```python
from build123d import *

# Parameters (mm, degrees)
F0_W      = 67.6028169692
F0_H      = 53.0741475523
F1_DEPTH  = 37.4
F2_R      = 11.3511276649
F2_R_2    = 7.9567380282
F3_DEPTH  = 6.7
F4_R      = 4.4090907082
F4_R_2    = 5.1686616875
F5_DEPTH  = 3.4
F7_DEPTH  = 2.1
F8_W      = 34.6914194524
F8_H      = 6.529385224
F9_DEPTH  = 4.6
F10_W     = 88.7872502208
F10_H     = 44.3032570183
F11_DEPTH = 87.7
F12_W     = 22.9829689488
F12_H     = 93.6014018953
F13_DEPTH = 18.4
F14_W     = 23.3173291199
F14_H     = 77.2590063095
F14_H_2   = 16.0102971315
F15_DEPTH = 18.6
F16_W     = 27.0305555314
F16_H     = 14.4476275891
F16_W_2   = 26.7750890926
F16_H_2   = 15.4520794749
F17_DEPTH = 103
F18_W     = 27.0305555314
F18_H     = 29.6849496663
F18_W_2   = 28.8268793374
F19_DEPTH = 10
F20_R     = 5


with BuildPart() as f1:
    # F0 (on Front) → F1 (new body)
    with BuildSketch(Plane.XZ):
        with Locations((1.2461747974, -5.0753373653)):
            Rectangle(F0_W, F0_H)
    extrude(amount=F1_DEPTH)

    # F2 (on face) → F3 (join)
    with BuildSketch(Plane.XZ.offset(37.4)):
        with Locations((-14.182465151, 1.8661138602)):
            Circle(F2_R)
        with Locations((17.3548590392, 0)):
            Circle(F2_R_2)
    extrude(amount=F3_DEPTH)

    # F4 (on face) → F5 (cut)
    with BuildSketch(Plane.XZ.offset(44.1)):
        with Locations((-14.182465151, 1.8661138602)):
            Circle(F4_R)
        with Locations((17.1402301639, 0)):
            Circle(F4_R_2)
    extrude(amount=-F5_DEPTH, mode=Mode.SUBTRACT)

    # F6 (on face) → F7 (cut)
    with BuildSketch(Plane.XZ.offset(37.4)):
        with BuildLine():
            add(Edge.make_bspline(
                [(-21.2736967951, -12.5029627234), (-17.6056978222, -10.7879533319), (1.7937398343, -27.2198277591), (39.0741519283, -6.345360962), (7.1844121531, -32.2427894232), (-23.5988764514, -26.0051011351), (-23.4195291506, -13.5062679776), (-21.2736967951, -12.5029627234)],
                knots=[0, 0, 0, 0, 0.217341047, 0.4323199028, 0.6402459683, 0.8728523496, 1, 1, 1, 1], degree=3))
        make_face()
    extrude(amount=-F7_DEPTH, mode=Mode.SUBTRACT)

    # F8 (on face) → F9 (join)
    with BuildSketch(Plane(origin=(0, 0, -31.6124111414), x_dir=(1, 0, 0), z_dir=(0, 0, -1))):
        with Locations((2.0386911929, 19.4482291117)):
            Rectangle(F8_W, F8_H)
    extrude(amount=F9_DEPTH)

    # F10 (on face) → F11 (join)
    with BuildSketch(Plane(origin=(0, 0, -36.2124111414), x_dir=(1, 0, 0), z_dir=(0, 0, -1))):
        with Locations((0.4012212157, 17.9098602384)):
            Rectangle(F10_W, F10_H)
    extrude(amount=F11_DEPTH)

    # F12 (on face) → F13 (join)
    with BuildSketch(Plane.YZ.offset(44.7948463261)):
        with Locations((-18.3663782664, -93.6325211078)):
            Rectangle(F12_W, F12_H)
    extrude(amount=F13_DEPTH)

    # F14 (on face) → F15 (join)
    with BuildSketch(Plane(origin=(-43.9924038947, 0, 0), x_dir=(0, -1, 0), z_dir=(-1, 0, 0))):
        with Locations((18.3590447996, -85.2829079866)):
            Rectangle(F14_W, F14_H)
        with Locations((18.3590447996, -131.9175597072)):
            Rectangle(F14_W, F14_H_2)
    extrude(amount=F15_DEPTH)

    # F16 (on face) → F17 (join)
    with BuildSketch(Plane(origin=(0, 0, -123.9124111414), x_dir=(1, 0, 0), z_dir=(0, 0, -1))):
        with Locations((-13.5152777657, 15.4278827831)):
            Rectangle(F16_W, F16_H)
        with Locations((22.6432844065, 15.930108726)):
            Rectangle(F16_W_2, F16_H_2)
    extrude(amount=F17_DEPTH)

    # F18 (on face) → F19 (join)
    with BuildSketch(Plane(origin=(0, 0, -226.9124111414), x_dir=(1, 0, 0), z_dir=(0, 0, -1))):
        with Locations((-13.5152777657, 23.0465438217)):
            Rectangle(F18_W, F18_H)
        with Locations((21.6039149091, 23.0465438217)):
            Rectangle(F18_W_2, F18_H)
    extrude(amount=F19_DEPTH)

    # F20
    f20_edges = [f1.edges().sort_by_distance(p)[0] for p in [
        (-62.592404, -30.017709, -93.288057),
    ]]
    fillet(f20_edges, radius=F20_R)


solid = f1.part
```
Could you check a few things on this model? Use its own coordinates, in mm. A direction names the side the tool comes from. Round coordinates to 2 decimals unless told otherwise and drop trailing zeros. Write each loop counter-clockwise with the first axis right and the second up, starting at its lowest first coordinate (ties: lowest second). Pieces come first, ordered by that corner, then holes. Notation, with made-up numbers: M -38,38 L -17,38 A18 ccw -17,50 Z; hole C -17.5,47.25 d7. An arc over 180 degrees is marked long. Write each question's results on one line, items separated by ' | '. Start each with the question number.
1. Thinking about a two-plate mould opening in Z: for faces 1 (the face through (21, -37.889, -232)), 2 (the face through (-53, -18, -46.653)), 3 (the face through (2, -22.713, -34)), 4 (the face through (17, -40.7, 0)), which applies, +Z half, -Z half, draft (parallel to the pull), parting line (faces both ways), or undercut?
2. I'm going to push flat-ended pins straight in: pin 1 Ø12.5 at (y, z) = (-17.5, -179) entering from -X; pin 2 Ø5.5 at (x, z) = (-51, -75.5) entering from +Y; pin 3 Ø11 at (y, z) = (-22, 1) entering from +X; pin 4 Ø5 at (y, z) = (-28.5, -178.5) entering from -X. Where does each tip first touch, or does it pass through?
3. Imagine slicing it at C-C on z = -94.5. List the corners of the cut face in (x, y) for me, and give its area (3 significant figures).
4. Imagine slicing it at D-D on x = -48.5. List the corners of the cut face in (y, z) for me, and give its area (3 significant figures).
5. On a 3-axis mill with a long thin cutter (end or side, diameter ignored), from which of +Z, -Z, +X, -X, +Y, -Y can I reach the whole of each face in a straight line? I mean faces 5 (the face through (54, -6.875, -94)), 6 (the face through (2, -16.184, -34)), 7 (the face through (1, 0, -5)), 8 (the face through (36.017, -23, -232)). Say none if no direction works.
6. I need wall thicknesses on L1, parallel to Z at x = -6, y = -25.5; L2, parallel to Z at x = -2, y = -13.5; L3, parallel to Z at x = 6, y = -13.5. Which ranges of each line are inside material? Lowest first, please. Write a range as from..to.
7. Imagine slicing it at B-B on z = -169.5. List the corners of the cut face in (x, y) for me, and give its area (3 significant figures).
Result sheet:
1) face 1: draft | face 2: +Z half | face 3: undercut | face 4: undercut
2) pin 1: stops at x = -27.03 | pin 2: stops at y = -6.7 | pin 3: stops at x = 35.05 | pin 4: passes through
3) outline: M -62.59,-25.02 A5 ccw -57.59,-30.02 L -43.99,-30.02 L -43.99,-40.06 L 44.79,-40.06 L 44.79,-29.86 L 63.19,-29.86 L 63.19,-6.87 L 44.79,-6.87 L 44.79,4.24 L -43.99,4.24 L -43.99,-6.7 L -62.59,-6.7 Z | area: 4,780 mm^2
4) outline: M -30.02,-139.92 L -6.7,-139.92 L -6.7,-46.65 L -30.02,-46.65 Z | area: 2,170 mm^2
5) face 5: +Z, -Z, +X, +Y | face 6: +X, -X, +Y | face 7: +Z, +X, -X, +Y | face 8: -Z, +X, +Y, -Y
6) L1: z = -236.91..-226.91, -123.91..-36.21, -31.61..21.46 | L2: z = -236.91..-36.21, -31.61..21.46 | L3: z = -123.91..-36.21, -31.61..21.46
7) outline: M -27.03,-22.65 L 0,-22.65 L 0,-8.2 L -27.03,-8.2 Z; M 9.26,-23.66 L 36.03,-23.66 L 36.03,-8.2 L 9.26,-8.2 Z | area: 804 mm^2
